```python
from build123d import *

# Parameters (mm, degrees)
F0_W     = 41.9582277536
F0_H     = 96.0698723793
F1_DEPTH = 45.72
F2_DEPTH = 47.244
F3_R     = 27.0129618135
F3_R_2   = 19.972912416
F4_DEPTH = 25.4
F5_DEPTH = 76.708


with BuildPart() as f1:
    # F0 (on Right) → F1 (new body)
    with BuildSketch(Plane.YZ):
        Rectangle(F0_W, F0_H)
    extrude(amount=F1_DEPTH)

    # F2 (add): a face of the model
    f2_faces = [f1.faces().sort_by_distance(p)[0] for p in [
        (0, 0, 0),
    ]]
    extrude(f2_faces, amount=F2_DEPTH)

    # F3 (on face) → F4 (join)
    with BuildSketch(Plane.XZ.offset(20.9791138768)):
        Circle(F3_R)
        Circle(F3_R_2, mode=Mode.SUBTRACT)
    extrude(amount=F4_DEPTH)

    # F5 (cut): a face of the model
    f5_faces = [f1.faces().sort_by_distance(p)[0] for p in [
        (0, -20.9791138768, 0),
    ]]
    extrude(f5_faces, amount=-F5_DEPTH, mode=Mode.SUBTRACT)


solid = f1.part
```
Can you work these out from the model? Positions are in its coordinate system, mm. A direction names the side the tool comes from. Round coordinates to 2 decimals unless told otherwise and drop trailing zeros. Loops run counter-clockwise (first coordinate to the right, second up) from the corner with the lowest first, then second, coordinate; pieces in that order, holes last. Notation, with made-up numbers: M -25,41.5 L -13,41.5 A14 ccw -13,46.5 Z; hole C 2,19.25 d3. An arc over 180 degrees is marked long. Answer as a JSON object with one key per item and string values. Group by question number.
Q1. Imagine slicing it at A-A, the plane x = 0. Please give me the cut outline in (y, z), then the cut area to 3 significant figures.
Q2. Imagine slicing it at D-D, the plane x = 24. Please give me the cut outline in (y, z), then the cut area to 3 significant figures.
Q3. On a 3-axis mill with a long thin cutter (end or side, diameter ignored), from which of +Z, -Z, +X, -X, +Y, -Y can I reach the whole of each face in a straight line? I mean faces 1 (the flat face through (45.72, 0, 1)), 2 (the flat face through (21, -20.979, 21)). Say none if no direction works.
Q4. Imagine slicing it at C-C, the plane y = -8. Please give me the cut outline in (x, z).
Q5. Please list where these lines run through material, in increasing order: L1, parallel to Z at x = 0, y = -39.75; L2, parallel to Z at x = 0, y = 10; L3, parallel to Y at x = -33, z = 13.
Q6. Will these pins go through, and if not, where does the flat tip stop? pin 1 (1 mm diameter, centred on x = -34, z = -9.5, fed in from -Y); pin 2 (6 mm diameter, centred on y = -29.5, z = 10.5, fed in from -X); pin 3 (5 mm diameter, centred on x = 23, y = -30.5, fed in from +Z).
Q7. Imagine slicing it at B-B, the plane z = 0. Please give me the cut outline in (x, y).
Findings:
{
 "1": {"outline": "M -46.38,-27.01 L -20.98,-27.01 L -20.98,-48.03 L 20.98,-48.03 L 20.98,-19.97 L -46.38,-19.97 Z; M -46.38,19.97 L 20.98,19.97 L 20.98,48.03 L -20.98,48.03 L -20.98,27.01 L -46.38,27.01 Z", "area": "2,710 mm2"},
 "2": {"outline": "M -46.38,-12.4 L -20.98,-12.4 L -20.98,-48.03 L 20.98,-48.03 L 20.98,48.03 L -20.98,48.03 L -20.98,12.4 L -46.38,12.4 Z", "area": "4,660 mm2"},
 "3": {"face 1": "+Z, -Z, +X, +Y, -Y", "face 2": "-Y"},
 "4": {"outline": "M -47.24,-48.03 L 45.72,-48.03 L 45.72,48.03 L -47.24,48.03 Z; hole C 0,0 d39.95"},
 "5": {"L1": "z = -27.01 to -19.97, 19.97 to 27.01", "L2": "z = -48.03 to -19.97, 19.97 to 48.03", "L3": "y = -20.98 to 20.98"},
 "6": {"pin 1": "stops at y = -20.98", "pin 2": "stops at x = -25.95", "pin 3": "stops at z = 17.59"},
 "7": {"outline": "M -47.24,-20.98 L -27.01,-20.98 L -27.01,-46.38 L -19.97,-46.38 L -19.97,20.98 L -47.24,20.98 Z; M 19.97,-46.38 L 27.01,-46.38 L 27.01,-20.98 L 45.72,-20.98 L 45.72,20.98 L 19.97,20.98 Z"}
}
